CAD build for the part. Positions are in the model's coordinates, mm. A direction names the side the tool comes from. Coordinates: 2 decimals unless noted, no trailing zeros. Write each loop counter-clockwise with the first axis right and the second up, starting at its lowest first coordinate (ties: lowest second). Pieces come first, ordered by that corner, then holes. Notation, with made-up numbers: (33, 33.25) - (51, 33.25) arc R15 ccw to (51, 50.25) - close; hole circle Ø3 at (87.25, -31.75). An arc over 180 degrees is marked (long way). One line per question, with ' | ' between items. Start each with the question number.
1. Which spindle directions (+Z, -Z, +X, -X, +Y, -Y) get a long thin tool onto all of the face, cutting with end or side? Do faces 5 (the cylindrical face through (11.61, 7.47, 3.62)), 6 (the flat face through (10.1, 6.8, -41.5)), 7 (the flat face through (10, 39.9, -20)). Say none if no direction does.
2. Band-saw the part on D-D, the plane y = 4.5. Write the cut outline in (x, z).
3. Two-plate mould, pull along X, no slides. Class faces 1 (the cylindrical face through (9.95, 36.25, -4.06)), 2 (the cylindrical face through (10, 9, -44)), 3 (the flat face through (13.2, 10.1, 1.5)), 4 (the flat face through (6.75, -2, -31)): +X half, -X half, draft (parallel to the pull), parting line (faces both ways), or undercut.
4. Band-saw the part on C-C, the plane z = -1.5. Write the cut outline in (x, y).
5. Band-saw the part on A-A, the plane z = -35.5. Write the cut outline in (x, y).
6. Flat gauge pins, fed straight in: P1, Ø2, axis at x = 10, y = 25, coming from the +Z side; P2, Ø2, axis at x = 10, y = 10, coming from the +Z side; P3, Ø4, axis at x = 17.5, y = 37.5, coming from the -Z side. Where does each tip first touch, or does it go through?
7. Band-saw the part on B-B, the plane y = 32. Write the cut outline in (x, z), then the cut area to 3 significant figures.
8. Probe line 1 (X direction, y = 37.5, z = -34); line 2 (Y direction, x = 2.5, z = -34.75); line 3 (Y direction, x = 10, z = -3). List the from-to ranges inside material, lowest first.
Autodesk Inventor part; units mm, degrees
ref_plane "YZ Plane" through (0, 0, 0) normal (1, 0, 0) x (0, 1, 0)
ref_plane "XZ Plane" through (0, 0, 0) normal (0, 1, 0) x (-1, 0, 0)
ref_plane "XY Plane" through (0, 0, 0) normal (0, 0, 1) x (1, 0, 0)
sketch "スケッチ1" plane through (0, 0, 0) normal (1, 0, 0) x (0, 1, 0)
  line L0 (0, 0) -> (40, 0)
  line L1 (40, 0) -> (40, -40)
  line L2 (40, -40) -> (0, -40)
  line L3 (0, -40) -> (0, 0)
  dimension "d0" = 40
  dimension "d1" = 40
extrude "押し出し1" add sketch "スケッチ1" along normal blind 20
sketch "スケッチ2" plane through (0, 0, 0) normal (0, 0, 1) x (1, 0, 0)
  circle A0 centre (10, 10) radius 7.5
  line L0 (0, 0) -> (20, 0)
  line L1 (0, 40) -> (0, 0)
  dimension "d4" = 15
  dimension "d5" = 10
  dimension "d6" = 10
extrude "押し出し2" add sketch "スケッチ2" along normal blind 1.5
sketch "スケッチ3" plane through (0, 0, -40) normal (0, 0, -1) x (-1, 0, 0)
  circle A0 centre (-10, 10) radius 7.5
  line L0 (0, 0) -> (-20, 0)
  line L1 (0, 0) -> (0, 40)
  dimension "d9" = 15
  dimension "d10" = 10
  dimension "d11" = 10
extrude "押し出し3" add sketch "スケッチ3" along normal blind 1.5
sketch "スケッチ4" plane through (20, 0, 0) normal (1, 0, 0) x (0, 0, -1)
  line L0 (40, 40) -> (0, 40)
  line L1 (20, 40) -> (20, 0)
  line L2 (0, 0) -> (40, 0)
  line L3 (11.5, 40) -> (28.5, 40)
  line L4 (28.5, 40) -> (28.5, 0)
  line L5 (28.5, 0) -> (11.5, 0)
  line L6 (11.5, 0) -> (11.5, 40)
  dimension "d14" = 17
extrude "押し出し4" cut sketch "スケッチ4" against normal blind 0.1
sketch "スケッチ5" plane through (0, 40, 0) normal (0, 1, 0) x (1, 0, 0)
  line L0 (0, 0) -> (0, 40)
  line L1 (0, 20) -> (19.9, 20)
  line L2 (19.9, 11.5) -> (19.9, 28.5)
  line L3 (19.9, 11.5) -> (0, 11.5)
  line L4 (0, 11.5) -> (0, 28.5)
  line L5 (0, 28.5) -> (19.9, 28.5)
  line L6 (19.9, 28.5) -> (19.9, 11.5)
extrude "押し出し5" cut sketch "スケッチ5" against normal blind 0.1
sketch "スケッチ6" plane through (0, 0, 0) normal (-1, 0, 0) x (0, 0, 1)
  line L0 (-11.5, 39.9) -> (-28.5, 39.9)
  line L1 (-20, 39.9) -> (-20, 0)
  line L2 (-28.5, 0) -> (-11.5, 0)
  line L3 (-28.5, 39.9) -> (-11.5, 39.9)
  line L4 (-11.5, 39.9) -> (-11.5, 0)
  line L5 (-11.5, 0) -> (-28.5, 0)
  line L6 (-28.5, 0) -> (-28.5, 39.9)
  point P0 (0, 0)
extrude "押し出し6" cut sketch "スケッチ6" against normal blind 0.1
sketch "スケッチ7" plane through (0, 0, -40) normal (0, -1, 0) x (1, 0, 0)
  line L0 (0.1, 28.5) -> (0.1, 11.5)
  line L1 (20, 28.5) -> (0, 28.5)
  line L2 (0.1, 11.5) -> (20, 11.5)
  line L3 (20, 11.5) -> (20, 28.5)
  line L4 (20, 28.5) -> (0.1, 28.5)
  line L5 (0.1, 28.5) -> (0.1, 11.5)
  point P0 (0, 40)
extrude "押し出し7" cut sketch "スケッチ7" against normal blind 0.1
sketch "スケッチ8" plane through (0, 0, -40) normal (0, 0, -1) x (-1, 0, 0)
  line L0 (0, 40) -> (-20, 40)
  line L1 (-20, 0) -> (-20, 40)
  line L2 (0, 0) -> (0, 40)
  point P0 (-17.5, 37.5)
  point P1 (-2.5, 37.5)
  point P2 (-2.5, 22.5)
  point P3 (-17.5, 22.5)
  dimension "d23" = 2.5
  dimension "d24" = 2.5
  dimension "d25" = 2.5
  dimension "d26" = 15
hole "穴1" at (17.5, 37.5, -40) at (2.5, 37.5, -40) at (2.5, 22.5, -40) at (17.5, 22.5, -40) direction (0, 0, 1) diameter 2.5 depth 8 tip angle 118
sketch "スケッチ9" plane through (0, 0, 0) normal (0, 0, 1) x (1, 0, 0)
  line L0 (0, 40) -> (20, 40)
  line L1 (20, 40) -> (20, 0)
  line L2 (0, 40) -> (0, 0)
  circle A0 centre (10, 30) radius 5
  point P0 (10, 25)
  point P1 (5, 30)
  point P2 (15, 30)
  point P3 (10, 35)
  dimension "d48" = 10
  dimension "d49" = 10
  dimension "d50" = 10
hole "穴2" at (10, 25, 0) at (5, 30, 0) at (15, 30, 0) at (10, 35, 0) direction (0, 0, -1) diameter 2.5 depth 8 tip angle 118
sketch "スケッチ10" plane through (10, 10, 1.5) normal (0, 0, 1) x (1, 0, 0)
  circle A0 centre (0, 0) radius 7.5
  circle A1 centre (0, 0) radius 3
  point P0 (-10, -10)
  dimension "d45" = 6
extrude "押し出し8" add sketch "スケッチ10" along normal blind 4.3 contours A1
sketch "スケッチ11" plane through (10, 10, -41.5) normal (0, 0, -1) x (-1, 0, 0)
  circle A0 centre (0, 0) radius 7.5
  circle A1 centre (0, 0) radius 3
  circle A2 centre (0, 0) radius 1
  point P0 (10, -10)
  dimension "d51" = 6
  dimension "d54" = 2
extrude "押し出し9" add sketch "スケッチ11" along normal blind 5.5 contours A1
sketch "スケッチ12" plane through (0, 0, -40) normal (0, -1, 0) x (1, 0, 0)
  line L0 (20, 11.5) -> (0, 11.5)
  line L1 (13.25, 11.5) -> (6.75, 11.5)
  line L2 (6.75, 11.5) -> (6.75, 7)
  line L3 (6.75, 7) -> (13.25, 7)
  line L4 (13.25, 7) -> (13.25, 11.5)
  point P0 (0, 40)
  point P1 (6.75, 11.5)
  point P2 (10, 11.5)
  dimension "d55" = 6.5
  dimension "d56" = 4.5
extrude "押し出し10" add sketch "スケッチ12" along normal blind 5
sketch "スケッチ13" plane through (10, 10, 5.8) normal (0, 0, 1) x (1, 0, 0)
  point P0 (0, 0)
hole "穴3" at (10, 10, 5.8) direction (0, 0, -1) diameter 2.459 depth 8 tip angle 120
properties part number "サーボモーター25kgcmサーボモータ" material "アルミニウム 6061"
Filled in:
1) face 5: +Z | face 6: -Z | face 7: +X, -X, +Y
2) outline: (0, -40) - (4.9, -40) - (4.9, -41.5) - (15.1, -41.5) - (15.1, -40) - (20, -40) - (20, -28.5) - (19.9, -28.5) - (19.9, -11.5) - (20, -11.5) - (20, 0) - (15.1, 0) - (15.1, 1.5) - (4.9, 1.5) - (4.9, 0) - (0, 0) - (0, -11.5) - (0.1, -11.5) - (0.1, -28.5) - (0, -28.5) - close
3) face 1: undercut | face 2: undercut | face 3: draft | face 4: -X half
4) outline: (0, 0) - (20, 0) - (20, 40) - (0, 40) - close; hole circle Ø2.5 at (5, 30); hole circle Ø2.5 at (10, 25); hole circle Ø2.5 at (10, 35); hole circle Ø2.46 at (10, 10); hole circle Ø2.5 at (15, 30)
5) outline: (0, 0) - (20, 0) - (20, 40) - (0, 40) - close; hole circle Ø2.5 at (2.5, 22.5); hole circle Ø2.5 at (2.5, 37.5); hole circle Ø2.5 at (17.5, 22.5); hole circle Ø2.5 at (17.5, 37.5)
6) P1: stops at z = -8.15 | P2: stops at z = -2.33 | P3: stops at z = -40
7) outline: (0, -40) - (20, -40) - (20, -28.5) - (19.9, -28.5) - (19.9, -11.5) - (20, -11.5) - (20, 0) - (0, 0) - (0, -11.5) - (0.1, -11.5) - (0.1, -28.5) - (0, -28.5) - close | area: 797 mm²
8) line 1: x = 0 to 1.25, 3.75 to 16.25, 18.75 to 20 | line 2: y = 0 to 21.25, 23.75 to 36.25, 38.75 to 40 | line 3: y = 0 to 23.75, 26.25 to 33.75, 36.25 to 40
